Input: part model. Units: mm. Frame: model coordinates. A direction names the side the tool comes from. Coordinates: 2 decimals unless noted, no trailing zeros. Write each loop counter-clockwise with the first axis right and the second up, starting at its lowest first coordinate (ties: lowest second). Pieces come first, ordered by that corner, then holes. Notation, with made-up numbers: (14, 6.25) - (36, 6.25) arc R12 ccw to (36, 21.25) - close; hole circle Ø3 at (-30, 77.5). An arc over 180 degrees is marked (long way). One line per question, with ' | ' between items. Start each with the question number.
1) Section query C-C on y = 2.95. Return loops of the section in (x, z), and give its area (3 significant figures).
2) Line query: line 1 (X direction, y = 1.3, z = -7.75); line 2 (X direction, y = 1.8, z = -14); line 3 (Y direction, x = 45.5, z = -14). Output: solid intervals per line, ascending.
3) First-contact query: P1, Ø3, axis at x = 18, z = -15, coming from the +Y side; P2, Ø1.6, axis at y = 1, z = -16.5, coming from the +X side; P3, Ø4, axis at x = -27, z = -8.3, coming from the +Y side; P4, Ø1.6, axis at x = 43, y = 1, coming from the -Z side. Flat tips, straight axial feed; report the tip coordinate or a pass-through.
4) Reachability of faces 5 (the flat face through (-1, 2, -12)), 6 (the flat face through (-29.5, 1, -17)), 7 (the flat face through (29.5, 1, -17)), 8 (the conical face through (7.95, 1.78, -6.94)) from +Z, -Z, +X, -X, +Y, -Y: full face, straight path, thin tool, end or side. Return the list, or none.
5) Section query B-B on x = 37.5. Return loops of the section in (y, z), and give its area (3 significant figures).
6) Draft query along Z for faces 1 (the flat face through (-1, 2, -2)), 2 (the conical face through (25.32, 1.78, -7.93)), 3 (the flat face through (-50, 1, -7)), 4 (the flat face through (40, 1, -15)). Return one class per face: released by +Z, released by -Z, zero draft, split by the parting line, or undercut.
7) Section query A-A on x = 27. Return loops of the section in (y, z).
Autodesk Inventor part; units mm, degrees
ref_plane "YZ Plane" through (0, 0, 0) normal (1, 0, 0) x (0, 1, 0)
ref_plane "XZ Plane" through (0, 0, 0) normal (0, 1, 0) x (-1, 0, 0)
ref_plane "XY Plane" through (0, 0, 0) normal (0, 0, 1) x (1, 0, 0)
sketch "Szkic1" plane through (0, 0, 0) normal (1, 0, 0) x (0, 1, 0)
  line L0 (0, 0) -> (2, -2)
  line L1 (2, -2) -> (2, -19)
  line L2 (2, -19) -> (0, -19)
  line L3 (0, -19) -> (0, -2)
  line L4 (0, -2) -> (0, 0)
  line L5 (0, -2) -> (2, -2)
  line L6 (2, -2) -> (4.3, -4.3)
  line L7 (4.3, -4.3) -> (2, -4.3)
  line L8 (2, -2) -> (4.3, -4.3)
  line L9 (4.3, -4.3) -> (2, -4.3)
  line L10 (4, -4) -> (4, -4.3) construction
  line L11 (4, -4) -> (2, -4) construction
  line L12 (4.3, -4.3) -> (4.3, -4.8)
  line L13 (4.3, -4.8) -> (2, -4.8)
  line L14 (0, 0) -> (-0.5, 0)
  line L15 (-0.5, 0) -> (-0.5, -19)
  line L16 (-0.5, -19) -> (0, -19)
  line L17 (0, -19) -> (0, 0)
  point P0 (5, -5)
  point P1 (4.3, -4.3)
  dimension "d1" = 2
  dimension "d2" = 45
  dimension "d44" = 45
  dimension "d45" = 2
  dimension "d46" = 17
  dimension "d50" = -4.3
  dimension "d51" = 19
  dimension "d54" = 0
  dimension "d98" = 2.3
  dimension "d125" = 4
  dimension "d126" = 0.3
  dimension "d156" = 0.5
  dimension "d157" = 0.5
extrude "Wyciągnięcie proste1" add sketch "Szkic1" along normal mid plane 100 contours L0 L5 L4 | L6 L7 L1 | L1 L2 L3 L5
sketch "Sketch4" plane through (-50, 0, -19) normal (0, -1, 0) x (1, 0, 0)
  line L0 (0, 0) -> (0, 19)
  line L1 (0, 0) -> (100, 0)
  line L2 (100, 19) -> (100, 0)
  line L3 (100, 19) -> (0, 19)
  line L4 (80, 0) -> (80, 19)
  line L5 (100, 19) -> (50, 19)
  line L6 (20, 19) -> (20, 0)
  line L7 (0, 0) -> (100, 0)
  line L8 (0, 14.7) -> (100, 14.7)
  circle A0 centre (77, 10.7) radius 3
  circle A1 centre (41, 10.7) radius 3
  circle A2 centre (23, 10.7) radius 3
  line L9 (80, 10.7) -> (20, 10.7)
  line L10 (80, 4) -> (20, 4)
  circle A3 centre (59, 10.7) radius 3
  circle A4 centre (68, 4) radius 3
  circle A5 centre (50, 4) radius 3
  circle A6 centre (32, 4) radius 3
  dimension "d67" = 6
  dimension "d70" = 6
  dimension "d22" = 20
  dimension "d23" = 20
  dimension "d69" = 6
  dimension "d75" = 18
  dimension "d127" = 6
  dimension "d129" = 18
  dimension "d139" = 18
  dimension "d140" = 6
  dimension "d141" = 6
  dimension "d142" = 6
  dimension "d143" = 9
  dimension "d144" = 9
  dimension "d145" = 9
  dimension "d146" = 9
  dimension "d147" = 9
  dimension "d148" = 9
  dimension "d149" = 4
  dimension "d150" = 4
hole "Hole2" at (27, 0, -8.3) at (-9, 0, -8.3) at (-27, 0, -8.3) at (9, 0, -8.3) at (0, 0, -15) at (18, 0, -15) at (-18, 0, -15) direction (0, 1, 0) diameter 3.2 depth 8.8 countersink diameter 7 countersink angle 90
extrude "Extrusion7" [suppressed]
sketch "Sketch5" plane through (-50, 0, 0) normal (0, -1, 0) x (1, 0, 0)
  line L0 (100, 0) -> (100, -19)
  line L1 (100, 0) -> (0, 0)
  line L2 (0, -19) -> (0, 0)
  line L3 (100, -15) -> (79.5, -15)
  line L4 (79.5, -15) -> (79.5, -32.132)
  line L5 (79.5, -32.132) -> (100, -32.132)
  line L6 (100, -32.132) -> (100, -15)
  line L7 (0, -19) -> (20.5, -19)
  line L8 (20.5, -19) -> (20.5, -15)
  line L9 (20.5, -15) -> (0, -15)
  line L10 (0, -15) -> (0, -19)
  circle A0 centre (23, -8.3) radius 3.5
  circle A1 centre (41, -8.3) radius 3.5
  circle A2 centre (77, -8.3) radius 3.5
  line L11 (0, -19) -> (100, -19)
  point P0 (50, 0)
  point P1 (0, -15)
  point P2 (100, -30)
  dimension "d55" = 20.5
  dimension "d56" = 20.5
  dimension "d61" = 15
  dimension "d62" = 15
extrude "Extrusion5" cut sketch "Sketch5" along normal through all both and the other way through all contours L0 L11 L4 L3 | L6 L5 L4 L11 | L9 L8 L7 L2
fillet "Fillet2" radius 1 2 edges at (-29.5, 1, -19) (29.5, 1, -19)
fillet "Fillet3" radius 1 2 edges at (-29.5, 1, -15) (29.5, 1, -15)
sketch "Sketch10" plane through (50, 0, 0) normal (1, 0, 0) x (0, 0, -1)
  line L0 (30.7582, 13.788) -> (30.3919, 3.2994)
  line L1 (30.5751, 8.5437) -> (-8.4118, 9.9052)
  line L2 (15, 0) -> (15, 2)
  line L3 (15, 2) -> (4.3, 2)
  line L4 (4.3, 2) -> (4.3, 4.3)
  line L5 (4.3, 4.3) -> (0, 0)
  line L6 (0, 0) -> (15, 0)
  line L7 (4.3, 2) -> (15, 2)
  line L8 (4.3, 2) -> (3.8, 2)
  circle A0 centre (63.2278, 12.35) radius 15
  line L9 (63.2278, 12.35) -> (63.2278, -2.65)
  line L10 (63.2278, -2.65) -> (0, 0)
  line L11 (0, 0) -> (0.1802, 4.3)
  line L12 (0.1802, 4.3) -> (3.8, 4.3)
  line L13 (3.8, 4.3) -> (3.8, 2)
  line L14 (3.8, 4.3) -> (4.3, 4.3) construction
  point P0 (3.8, 3.8)
  dimension "d166" = 90
  dimension "d167" = 0.5
extrude "Extrusion9" [suppressed]
sketch "Sketch11" plane through (50, 0, 0) normal (1, 0, 0) x (0, 0, -1)
  line L0 (3.8, 4.3) -> (3.8, 2)
  line L1 (4.3, 2) -> (3.8, 2)
  line L2 (4.3, 2) -> (4.3, 4.3)
  line L3 (4.3, 4.3) -> (0, 0)
  point P0 (3.8, 3.8)
extrude "Extrusion10" [suppressed]
sketch "Sketch12" plane through (-28.5, 0, -19) normal (0, -1, 0) x (1, 0, 0)
  arc A0 (57, 0) -> (58, 1) centre (57, 1) ccw
  line L0 (58, 1) -> (58, 3)
  arc A1 (59, 4) -> (58, 3) centre (59, 3) ccw
  line L1 (59, 4) -> (78.5, 4)
  line L2 (78.5, 19) -> (78.5, 4)
  line L3 (78.5, 19) -> (-21.5, 19)
  line L4 (-21.5, 4) -> (-21.5, 19)
  line L5 (-21.5, 4) -> (-2, 4)
  arc A2 (-1, 3) -> (-2, 4) centre (-2, 3) ccw
  line L6 (-1, 3) -> (-1, 1)
  arc A3 (-1, 1) -> (0, 0) centre (0, 1) ccw
  line L7 (0, 0) -> (57, 0)
  circle A4 centre (55.5, 10.7) radius 3.5
  circle A5 centre (19.5, 10.7) radius 3.5
  circle A6 centre (1.5, 10.7) radius 3.5
  circle A7 centre (37.5, 10.7) radius 3.5
  circle A8 centre (28.5, 4) radius 3.5
  circle A9 centre (46.5, 4) radius 3.5
  circle A10 centre (10.5, 4) radius 3.5
  arc A11 (57, 0.5) -> (57.5, 1) centre (57, 1) ccw
  line L8 (57.5, 1) -> (57.5, 3)
  arc A12 (59, 4.5) -> (57.5, 3) centre (59, 3) ccw
  line L9 (59, 4.5) -> (78, 4.5)
  line L10 (78, 4.5) -> (78, 18.5)
  line L11 (78, 18.5) -> (-21, 18.5)
  line L12 (-21, 18.5) -> (-21, 4.5)
  line L13 (-21, 4.5) -> (-2, 4.5)
  arc A13 (-0.5, 3) -> (-2, 4.5) centre (-2, 3) ccw
  line L14 (-0.5, 3) -> (-0.5, 1)
  arc A14 (-0.5, 1) -> (0, 0.5) centre (0, 1) ccw
  line L15 (0, 0.5) -> (57, 0.5)
  line L16 (57, 0.5) -> (57.866, 0.5)
  line L17 (0, 0.5) -> (-0.866, 0.5)
  point P0 (28.5, 19)
  dimension "d172" = 0.5
extrude "Extrusion11" [suppressed]
fillet "Fillet4" [suppressed]
equation "\"d23\" = d22"
equation "\"d56\" = d55"
equation "\"d62\" = d61"
equation "\"d64\" = d80"
equation "\"d79\" = d64"
properties part number "Plog2" material "Steel, Carbon"
Answer key:
1) outline: (-50, -4.3) - (50, -4.3) - (50, -2.95) - (-50, -2.95) - close | area: 135 mm²
2) line 1: -50 to -29.13, -24.87 to -11.13, -6.87 to 6.87, 11.13 to 24.87, 29.13 to 50 | line 2: -50 to -19.37, -16.63 to -1.37, 1.37 to 16.63, 19.37 to 50 | line 3: 0 to 2
3) P1: through | P2: x = 29.55 | P3: y = 2 | P4: z = -15
4) face 5: -Z, +X, -X, +Y | face 6: -Z, -X, +Y, -Y | face 7: -Z, +X, +Y, -Y | face 8: -Y
5) outline: (0, -15) - (2, -15) - (2, -4.3) - (4.3, -4.3) - (0, 0) - close | area: 30.6 mm²
6) face 1: released by +Z | face 2: undercut | face 3: zero draft | face 4: released by -Z
7) outline: (0, -19) - (2, -19) - (2, -9.9) - (1.9, -9.9) - (0, -11.8) - close; (0, -4.8) - (1.9, -6.7) - (2, -6.7) - (2, -4.3) - (4.3, -4.3) - (0, 0) - close
